Read the model definition and answer for the solid it produces. Units are mm, in the model's axes. A direction names the side the tool comes from. Coordinates: 2 decimals unless noted, no trailing zeros. Order: outer loops, then holes, each group sorted by start corner. A loop starts at its lowest first (then second) coordinate and runs counter-clockwise, first axis right, second up. Notation, with made-up numbers: M -31,-27 L -25,-27 A11 cw -25,-8 Z; hole C 36,67.5 d8. An arc over 180 degrees is marked long. Use a Markdown table: item, result. Add a question column.
1) Find section C-C on y = 1.5. Count the separate pieces of the cut face and the enclosed holes in it, plus the area to 3 significant figures.
2) Find section D-D on z = 52.5. Write down the section's boundary in (x, y), plus the area to 3 significant figures.
3) Find section A-A on z = -21.5. Write down the section's boundary in (x, y).
4) Find section B-B on x = -5. Write down the section's boundary in (y, z), plus the area to 3 significant figures.
5) Find the intervals of material crossed by probe 1 along Z at (x, y) = (51.5, 1); probe 2 along Y at (x, z) = (53, 11); probe 3 along Z at (x, y) = (31, 1), in increasing order. Write a range as [from, to].
6) The mould has two halves that part along Z. Classify faces 4 (the face through (-31.01, 1.52, -11.7)), 5 (the face through (2.155, 1.521, -47.643)), 6 (the face through (-30.338, 1.479, 45.618)), 7 (the face through (46, 13, -4)): released by +Z, released by -Z, zero draft, split by the parting line, or undercut.
7) For faces 1 (the face through (15.741, 1, -56)), 2 (the face through (22, 3, -26)), 3 (the face through (56.885, 1.521, -5.219)), determine the directions among +Z, -Z, +X, -X, +Y, -Y from which every point of the face is accessible in a straight line to the end or side of a thin tool.
8) Each of these flat-tipped pins is pushed along its axis until it touches: pin 1 Ø6.5 at (x, z) = (37.49, 46.66) entering from +Y; pin 2 Ø3 at (y, z) = (6, 32.5) entering from -X; pin 3 Ø4.5 at (x, z) = (9.51, -59.15) entering from -Y; pin 4 Ø2.5 at (x, z) = (51.51, 30.95) entering from -Y. Where does it stop, or does it pass through?
from build123d import *

# Parameters (mm, degrees)
SKETCH4_R           = 36
BOSS_EXTRUDE1_DEPTH = 3
SKETCH5_R           = 2
SKETCH5_R_2         = 2.5
CUT_EXTRUDE1_DEPTH  = 93.694705096
CUT_EXTRUDE2_DEPTH  = 93.694705096
FILLET1_R           = 5
FILLET2_RADIUS      = 6.234464512
FILLET2_LENGTH      = 3
BOSS_EXTRUDE2_DEPTH = 10
FILLET4_START       = 3
FILLET4_DEPTH       = 11
FILLET5_START       = 3
FILLET5_DEPTH       = 11


with BuildPart() as part:
    # Sketch4 → Boss-Extrude1 (new body)
    with BuildSketch(Plane(origin=(0, 0, 0), x_dir=(1, 0, 0), z_dir=(0, 1, 0))):
        with BuildLine():
            Line((3.272204442, 66.499609121), (15.741133466, 66.499609121))
            Line((15.741133466, 66.499609121), (15.741133466, 46.499609121))
            ThreePointArc((15.741133466, 46.499609121), (9.506668954, -63.145898034), (3.272204442, 46.499609121))
            Line((3.272204442, 46.499609121), (3.272204442, 66.499609121))
        make_face()
        with Locations(Location((9.506668954, -8.145898034, 0), (0, 0, 270))):
            Circle(SKETCH4_R, mode=Mode.SUBTRACT)
    extrude(amount=BOSS_EXTRUDE1_DEPTH)

    # Sketch5 → Cut-Extrude1 (cut, through all)
    with BuildSketch(Plane(origin=(0, 3, 0), x_dir=(1, 0, 0), z_dir=(0, 1, 0))):
        with Locations(Location((9.506668954, 59.145898034, 0), (0, 0, 270))):
            Circle(SKETCH5_R)
        with Locations(Location((9.506668954, 39.454101966, 0), (0, 0, 270))):
            Circle(SKETCH5_R_2)
        with Locations(Location((54.77695913, 6.563310898, 0), (0, 0, 270))):
            Circle(SKETCH5_R_2)
        with Locations(Location((51.506668954, -30.947448364, 0), (0, 0, 270))):
            Circle(SKETCH5_R)
        with Locations(Location((37.485246963, -46.655106966, 0), (0, 0, 270))):
            Circle(SKETCH5_R_2)
        with Locations(Location((-18.471909055, -46.655106966, 0), (0, 0, 270))):
            Circle(SKETCH5_R_2)
        with Locations(Location((-32.493331046, -30.947448364, 0), (0, 0, 270))):
            Circle(SKETCH5_R_2)
        with Locations(Location((-33.116843335, 13.043632404, 0), (0, 0, 270))):
            Circle(SKETCH5_R_2)
    extrude(amount=-CUT_EXTRUDE1_DEPTH, mode=Mode.SUBTRACT)

    # Sketch6 → Cut-Extrude2 (cut, through all)
    with BuildSketch(Plane(origin=(0, 3, 0), x_dir=(1, 0, 0), z_dir=(0, 1, 0))):
        with BuildLine():
            Line((-31.240982332, -33.111154143), (-30.281144407, -54.888863669))
            Line((-30.281144407, -54.888863669), (-55.634525549, -56.00629692))
            Line((-55.634525549, -56.00629692), (-56.656818195, -8.246358342))
            Line((-56.656818195, -8.246358342), (-42.942031477, -7.625931476))
            ThreePointArc((-42.942031477, -7.625931476), (-34.312049589, -11.478197503), (-32.241689114, -20.699376843))
            Line((-32.241689114, -20.699376843), (-32.493331046, -28.447448364))
            ThreePointArc((-32.493331046, -28.447448364), (-30.078867912, -30.299090611), (-31.240982332, -33.111154143))
        make_face()
    extrude(amount=-CUT_EXTRUDE2_DEPTH, mode=Mode.SUBTRACT)

    # Fillet1
    fillet1_edges = [part.edges().sort_by_distance(p)[0] for p in [
        (3.272204442, 1.5, -46.499609121),
        (15.741133466, 1.5, -46.499609121),
        (-30.686613079, 1.5, 45.689207416),
        (-45.491842696, 1.5, 7.741279342),
    ]]
    fillet(fillet1_edges, radius=FILLET1_R)

    # Fillet2: full round fillet: the end face becomes a half cylinder, R = half its width
    fillet2_face = Plane((9.506668954, 1.5, -66.499609121), x_dir=(0, 1, 0), z_dir=(0, 0, -1))  # on the end face: x along it, z out of the body
    fillet2_slab = fillet2_face.offset(-FILLET2_RADIUS / 2) * Box(FILLET2_LENGTH, 2 * FILLET2_RADIUS, FILLET2_RADIUS, mode=Mode.PRIVATE)  # the body's end, R deep
    fillet2_round = Plane((9.506668954, 1.5, -60.265144609), x_dir=(0, 0, -1), z_dir=(0, 1, 0)) * Cylinder(FILLET2_RADIUS, FILLET2_LENGTH, mode=Mode.PRIVATE)  # its axis R under the face
    add(fillet2_slab - fillet2_round, mode=Mode.SUBTRACT)

    # Sketch9 → Boss-Extrude2 (add)
    with BuildSketch(Plane(origin=(0, 3, 0), x_dir=(1, 0, 0), z_dir=(0, 1, 0))):
        with BuildLine():
            Line((-31.282982054, -3.998082872), (-28.266279427, -3.998082872))
            ThreePointArc((-28.266279427, -3.998082872), (46.288733159, 1.397673249), (-21.484606715, -30.135459931))
            Line((-21.484606715, -30.135459931), (-21.484606715, -34.988789689))
            ThreePointArc((-21.484606715, -34.988789689), (48.599268457, 4.214064106), (-31.282982054, -3.998082872))
        make_face()
    extrude(amount=BOSS_EXTRUDE2_DEPTH)

    # Fillet4: read off the stored shape, not the designer's step
    # Fillet4 outline → Fillet4 (cut)
    with BuildSketch(Plane(origin=(0, 0, 0), x_dir=(1, 0, 0), z_dir=(0, 1, 0)).offset(FILLET4_START)):
        with BuildLine():
            ThreePointArc((-21.484606715, -34.988789689), (-21.295327251, -35.205776633), (-21.104528575, -35.421428933))
            add(Edge.make_bspline(
                [(-21.104528575, -35.421428933), (-21.228279098, -35.282544315), (-21.3411007, -35.112745613), (-21.431423393, -34.910535387), (-21.484606706, -34.678162347), (-21.484606715, -34.423543707)],
                knots=[0, 0, 0, 0, 0, 0, 0.275825991, 0.275825991, 0.275825991, 0.275825991, 0.275825991, 0.275825991], degree=5, weights=[1, 0.889669603, 0.794555202, 0.714656797, 0.649974387, 0.600507972]))
            Line((-21.484606715, -34.423543707), (-21.484606715, -34.988789689))
        make_face()
        with BuildLine():
            Line((-21.484606715, -30.135459931), (-21.484606715, -34.423543707))
            add(Edge.make_bspline(
                [(-21.484606715, -34.423543707), (-21.484606746, -33.500313944), (-20.896716335, -32.737133887), (-19.98906503, -32.613765882), (-19.271618069, -32.968959182), (-18.864684854, -33.425658379)],
                knots=[0.275825991, 0.275825991, 0.275825991, 0.275825991, 0.275825991, 0.275825991, 1, 1, 1, 1, 1, 1], degree=5, weights=[0.600507972, 0.47063518, 0.445647986, 0.525546392, 0.710330397, 1]))
            ThreePointArc((-18.864684854, -33.425658379), (-20.22020098, -31.816833883), (-21.484606715, -30.135459931))
        make_face()
    extrude(amount=FILLET4_DEPTH, mode=Mode.SUBTRACT)

    # Fillet5: read off the stored shape, not the designer's step
    # Fillet5 outline → Fillet5 (cut)
    with BuildSketch(Plane(origin=(0, 0, 0), x_dir=(1, 0, 0), z_dir=(0, 1, 0)).offset(FILLET5_START)):
        with BuildLine():
            ThreePointArc((-28.266279427, -3.998082872), (-28.19006415, -3.354623327), (-28.102888392, -2.712556866))
            add(Edge.make_bspline(
                [(-28.102888392, -2.712556866), (-28.151775573, -3.050953664), (-28.302840716, -3.42403045), (-28.598328595, -3.773471224), (-29.047777864, -3.998082872), (-29.587476182, -3.998082872)],
                knots=[0, 0, 0, 0, 0, 0, 0.464069746, 0.464069746, 0.464069746, 0.464069746, 0.464069746, 0.464069746], degree=5, weights=[1, 0.814372102, 0.671816349, 0.572332742, 0.515921281, 0.502581966]))
            Line((-29.587476182, -3.998082872), (-28.266279427, -3.998082872))
        make_face()
        with BuildLine():
            Line((-31.282982054, -3.998082872), (-29.587476182, -3.998082872))
            add(Edge.make_bspline(
                [(-29.587476182, -3.998082872), (-30.247519863, -3.998082872), (-30.77941952, -3.674118257), (-31.063082194, -3.179978591), (-31.130586894, -2.688704223), (-31.072063972, -2.283608879)],
                knots=[0.464069746, 0.464069746, 0.464069746, 0.464069746, 0.464069746, 0.464069746, 1, 1, 1, 1, 1, 1], degree=5, weights=[0.502581966, 0.487177078, 0.529216438, 0.628700044, 0.785627898, 1]))
            ThreePointArc((-31.072063972, -2.283608879), (-31.186553224, -3.13973496), (-31.282982054, -3.998082872))
        make_face()
    extrude(amount=FILLET5_DEPTH, mode=Mode.SUBTRACT)


solid = part.part
Check result:
| question | item | result |
|---|---|---|
| 1 | separate pieces | 1 |
| 1 | enclosed holes | 8 |
| 1 | area | 5,210 mm2 |
| 2 | outline | M -23.02,0 L 42.03,0 L 42.03,3 L -23.02,3 Z |
| 2 | area | 195 mm2 |
| 3 | outline | M -36.82,0 L -10.92,0 L -10.92,3 L -14.27,3 L -14.27,13 L -18.82,13 L -18.82,3 L -36.82,3 Z; M 29.93,0 L 55.83,0 L 55.83,3 L 37.83,3 L 37.83,13 L 33.28,13 L 33.28,3 L 29.93,3 Z |
| 4 | outline | M 0,-44.91 L 3,-44.91 L 3,-30.2 L 13,-30.2 L 13,-26.98 L 3,-26.98 L 3,-24.8 L 0,-24.8 Z; M 0,41.09 L 3,41.09 L 3,43.27 L 13,43.27 L 13,46.49 L 3,46.49 L 3,61.2 L 0,61.2 Z |
| 4 | area | 185 mm2 |
| 5 | probe 1 | z = [-27.37, 28.95], [32.95, 43.66] |
| 5 | probe 2 | y = [0, 3] |
| 5 | probe 3 | z = [-42.48, -20.73], [37.03, 58.77] |
| 6 | face 4 | undercut |
| 6 | face 5 | released by -Z |
| 6 | face 6 | released by +Z |
| 6 | face 7 | zero draft |
| 7 | face 1 | -Z, +X, +Y, -Y |
| 7 | face 2 | +Y |
| 7 | face 3 | +Y, -Y |
| 8 | pin 1 | stops at y = 3 |
| 8 | pin 2 | stops at x = -21.42 |
| 8 | pin 3 | stops at y = 0 |
| 8 | pin 4 | passes through |
